Solid Edge part; units mm, degrees
sketch "Sketch1" plane through (0, 0, 0) normal (0, 0, 1) x (1, 0, 0)
  line L0 (-28.8675, -16.6667) -> (28.8675, -16.6667)
  line L1 (28.8675, -16.6667) -> (0, 33.3333)
  line L2 (0, 33.3333) -> (-28.8675, -16.6667)
extrude "Protrusion1" add sketch "Sketch1" along normal blind 113.4955
sketch "Sketch2" plane through (0, 0, 0) normal (1, 0, 0) x (0, 1, 0)
  line L0 (-16.6667, 0) -> (0, 47.1405)
extrude "Cutout1" cut sketch "Sketch2" along normal up to next and the other way up to next material side at (0, -8.3805, 23.5869)
pattern_circular "Pattern1" count 3 over 360 about axis through (0, 0, 0) along (0, 0, 1) of "Cutout1"
The listing builds one solid part. Answer for the finished solid, in the listing's coordinates (mm). Give positions to 0.01 mm unless a question says otherwise; leave off trailing zeros. Write each loop counter-clockwise with the first axis right and the second up, starting at its lowest first coordinate (ties: lowest second). Pieces come first, ordered by that corner, then holes.
Item 1: Section B-B, the plane z = 29.5 is taken. Write down the section's boundary in (x, y).
Item 2: Section C-C, the plane y = -6 is taken. Write down the section's boundary in (x, z).
Item 3: Find the intervals of material crossed by line 1 along X through (y, z) = (-4, 5); line 2 along Z through (x, y) = (20, -2); line 3 along Z through (x, y) = (12, -4), in increasing order.
Item 4: Section A-A, the plane x = -15 is taken. Write down the section's boundary in (y, z).
Item 5: Flat-ended cylindrical pins translate along their axes: P1, Ø10, axis at y = -0.5, z = 23, coming from the +X side; P2, Ø5, axis at y = 7, z = 24, coming from the -X side; P3, Ø6, axis at y = -10.5, z = 24.5, coming from the -X side. Find the tip coordinate at first contact, or state that the pin passes through.
Completed:
1. outline: (-10.8, -6.24) - (10.8, -6.24) - (0, 12.47) - close
2. outline: (-22.71, 0) - (22.71, 0) - (10.39, 30.17) - (-10.39, 30.17) - close
3. line 1: x = -19.51 to 19.51
3. line 2: z = 0 to 0.98
3. line 3: z = 0 to 23.4
4. outline: (-16.67, 0) - (7.35, 0) - (-8.66, 22.65) - close
5. P1: stops at x = 13.68
5. P2: stops at x = -7.17
5. P3: stops at x = -15.42
